Autodesk Inventor part; units mm, degrees
ref_plane "YZ Plane" through (0, 0, 0) normal (1, 0, 0) x (0, 1, 0)
ref_plane "XZ Plane" through (0, 0, 0) normal (0, 1, 0) x (-1, 0, 0)
ref_plane "XY Plane" through (0, 0, 0) normal (0, 0, 1) x (1, 0, 0)
sketch "Sketch1" plane through (0, 0, 0) normal (0, 1, 0) x (-1, 0, 0)
  circle A0 centre (0, 0) radius 28
  line L0 (28, 0) -> (31.5, 0)
  circle A1 centre (0, 0) radius 31.5
  circle A2 centre (0, 0) radius 31.5
  circle A3 centre (0, 0) radius 31.5
  dimension "d0" = 56
  dimension "d1" = 3.5
extrude "Extrusion1" add sketch "Sketch1" along normal blind 13.25
sketch "Sketch2" plane through (0, 13.25, 0) normal (0, 1, 0) x (1, 0, 0)
  circle A0 centre (0, 0) radius 28
  line L0 (0, -28) -> (0, -24.5)
  line L1 (0, -24.5) -> (0, -31.5)
  circle A1 centre (0, 0) radius 31.5
  line L2 (0, -31.5) -> (0, -36)
  circle A2 centre (0, 0) radius 24.5
  circle A3 centre (0, 0) radius 36
  dimension "d4" = 3.5
  dimension "d5" = 4.5
extrude "Extrusion2" add sketch "Sketch2" along normal blind 3 contours A0 | A1 | A3
sketch "Sketch3" plane through (0, 0, 0) normal (0, -1, 0) x (1, 0, 0)
  circle A0 centre (0, 0) radius 31.5
  line L0 (0.0291, 31.5) -> (0.0291, -31.5)
  line L1 (2.8791, 31.3681) -> (2.8791, -35.492)
  line L2 (-2.8209, 31.3734) -> (-2.8209, -35.492)
  circle A1 centre (0, 0) radius 31.5
  circle A2 centre (0, 0) radius 30
  point P0 (2.8791, 29.8615)
  point P1 (2.8791, 31.3681)
  point P2 (-2.8209, 31.3734)
  point P3 (-2.8209, 29.8671)
  point P4 (2.8791, -29.8615)
  point P5 (-2.8209, -29.8671)
  point P6 (-2.8209, -31.3734)
  point P7 (2.8791, -31.3681)
  dimension "d8" = 2.85
  dimension "d9" = 2.85
extrude "Extrusion3" add sketch "Sketch3" along normal blind 5 contours L1 A2 L0 A0 | A0 L0 A2 L1 | L0 A2 L2 A0 | A0 L2 A2 L0
fillet "Fillet1" radius 1.5 2 edges at (-36, 13.25, 0) (-36, 16.25, 0)
properties part number "vez-rotate"
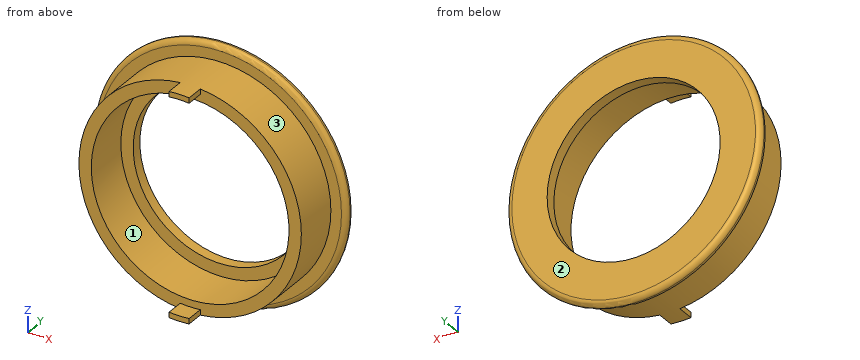
Input: part model. Units: mm. Frame: model coordinates. Face numbers are marked on the shaded views. Give positions to 0.01 mm unless a question says otherwise; leave off trailing zeros. Loops run counter-clockwise (first coordinate to the right, second up) from the corner with the lowest first, then second, coordinate; pieces in that order, holes last.
1) Section query A-A on y = -2. Return the cut outline in (x, z).
A:
outline: (-2.82, -31.37) arc R31.5 ccw to (2.88, -31.37) - (2.88, -29.86) arc R30 cw to (-2.82, -29.87) - close; (-2.82, 29.87) arc R30 cw to (2.88, 29.86) - (2.88, 31.37) arc R31.5 ccw to (-2.82, 31.37) - close
2) Section query D-D on y = 5.75. Return the cut outline in (x, z).
A:
outline: circle Ø63 at (0, 0); hole circle Ø56 at (0, 0)
3) Mould query, pull axis Z, two halves, no side actions, for the marked faces 1, 2 and 3. Classes: released by +Z, released by -Z, zero draft, split by the parting line, or undercut.
A:
face 1: undercut
face 2: zero draft
face 3: split by the parting line
4) Line query: L1, parallel to Z at x = 0, y = 9.25; L2, parallel to Y at x = -23.5, z = -21.5; L3, parallel to Z at x = 11, y = 1. Output: solid intervals per line, ascending.
A:
L1: z = -31.5 to -28, 28 to 31.5
L2: y = 13.25 to 16.25
L3: z = -29.52 to -25.75, 25.75 to 29.52
5) Contact query for flat-ended pins moving along their axis: pin 1 (5 mm diameter, centred on x = 10, y = 7.5, fed in from -Z); pin 2 (19 mm diameter, centred on x = 5.5, z = -13, fed in from -Y); pin 3 (8 mm diameter, centred on y = 0, z = 7.5, fed in from +X); pin 4 (10 mm diameter, centred on y = 4, z = -22.5, fed in from +X). Output: stop coordinate, or through.
A:
pin 1: stops at z = -30.59
pin 2: passes through
pin 3: stops at x = 31.3
pin 4: stops at x = 26.19
